Design review of the part built by this model. Coordinates are the model's own, in mm. Give positions to 0.01 mm unless a question says otherwise; leave off trailing zeros. Write each loop counter-clockwise with the first axis right and the second up, starting at its lowest first coordinate (ties: lowest second). Pieces come first, ordered by that corner, then holes.
```python
from build123d import *

# Parameters (mm, degrees)
F0_W     = 350
F0_H     = 40
F1_DEPTH = 20
F2_R     = 4
F3_DEPTH = 25
F4_R     = 4
F5_DEPTH = 25


with BuildPart() as f1:
    # F0 (on Front) → F1 (new body)
    with BuildSketch(Plane.XZ):
        Rectangle(F0_W, F0_H)
    extrude(amount=F1_DEPTH)

    # F2 (on face) → F3 (join)
    with BuildSketch(Plane.XZ.offset(20)):
        with Locations((-150, 0)):
            Circle(F2_R)
    extrude(amount=F3_DEPTH)

    # F4 (on face) → F5 (cut)
    with BuildSketch(Plane.XZ.offset(20)):
        with Locations((150, 0)):
            Circle(F4_R)
    extrude(amount=-F5_DEPTH, mode=Mode.SUBTRACT)


solid = f1.part
```
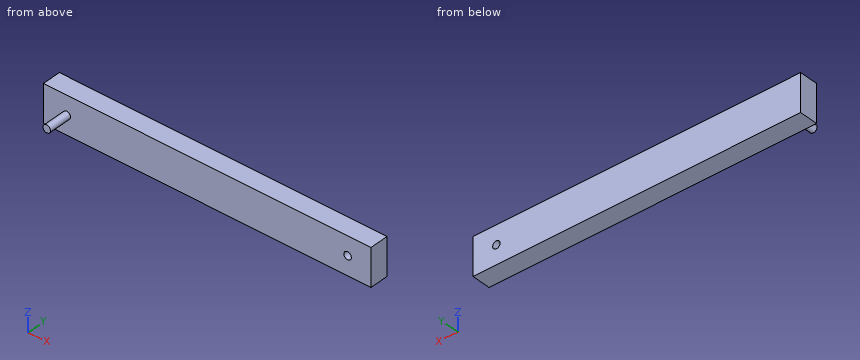
(1) Consider section A-A, the plane z = 0. Give the boundary of the cut face in (x, y).
Resolved:
outline: (-175, -20) - (-154, -20) - (-154, -45) - (-146, -45) - (-146, -20) - (146, -20) - (146, 0) - (-175, 0) - close; (154, -20) - (175, -20) - (175, 0) - (154, 0) - close
(2) To check wall thickness, follow L1, parallel to Z at x = 150, y = -7.25; L2, parallel to Y at x = -27, z = 17.5; L3, parallel to X at y = -13.5, z = -3.5. State the ranges of each line that lie inside material, in increasing order.
Resolved:
L1: z = -20 to -4, 4 to 20
L2: y = -20 to 0
L3: x = -175 to 148.06, 151.94 to 175
(3) Consider section C-C, the plane x = -150. Give the boundary of the cut face in (y, z).
Resolved:
outline: (-45, -4) - (-20, -4) - (-20, -20) - (0, -20) - (0, 20) - (-20, 20) - (-20, 4) - (-45, 4) - close
(4) Consider section D-D, the plane z = 16. Give the boundary of the cut face in (x, y).
Resolved:
outline: (-175, -20) - (175, -20) - (175, 0) - (-175, 0) - close
(5) Clearance check with flat-ended pins moving along their axes: P1, Ø10, axis at x = 80, y = -27, coming from the +Z side; P2, Ø20, axis at x = -47.5, z = -1, coming from the -Y side; P3, Ø4, axis at y = -23, z = 1.5, coming from the +X side. State where each tip first meets the part, or that it passes through.
Resolved:
P1: passes through
P2: stops at y = -20
P3: stops at x = -146
(6) Consider section B-B, the plane x = 150. Give the boundary of the cut face in (y, z).
Resolved:
outline: (-20, -20) - (0, -20) - (0, -4) - (-20, -4) - close; (-20, 4) - (0, 4) - (0, 20) - (-20, 20) - close
